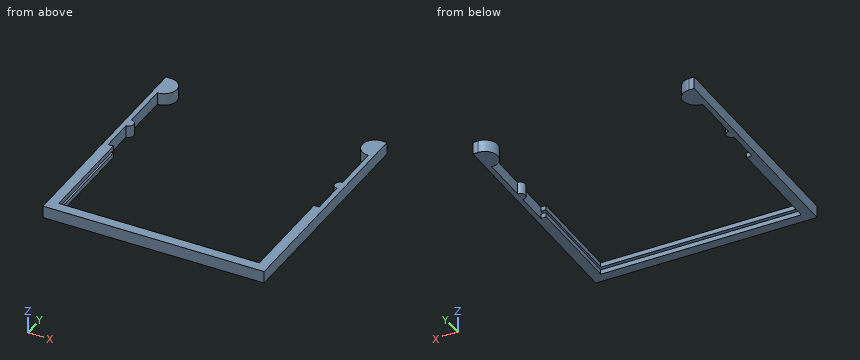
```python
from build123d import *

# Parameters (mm, degrees)
BOSS_EXTRUDE1_DEPTH      = 3
BOSS_EXTRUDE1_DEPTH_BACK = 3
CUT_EXTRUDE1_DEPTH       = 0.7
CUT_EXTRUDE1_DEPTH_BACK  = 0.7


with BuildPart() as part:
    # Sketch2 → Boss-Extrude1 (new body, two sides)
    with BuildSketch(Plane.XY) as boss_extrude1_sk:
        with BuildLine():
            Line((-52.1, 67.96), (-54.61, 67.96))
            Line((-54.61, 67.96), (-54.61, 9.929230009))
            Line((-54.61, 9.929230009), (-54.61, -46.34))
            Line((-54.61, -46.34), (54.61, -46.34))
            Line((54.61, -46.34), (54.61, 9.929230009))
            Line((54.61, 9.929230009), (54.61, 67.96))
            Line((54.61, 67.96), (52.1, 67.96))
            ThreePointArc((52.1, 67.96), (45.75, 61.61), (52.1, 55.26))
            Line((52.1, 55.26), (52.1, 43.8))
            Line((52.1, 43.8), (52.1, 31.2))
            ThreePointArc((52.1, 31.2), (49.6, 28.7), (52.1, 26.2))
            Line((52.1, 26.2), (52.1, 9.54))
            Line((52.1, 9.54), (49.53, 9.54))
            Line((49.53, 9.54), (49.53, -41.26))
            Line((49.53, -41.26), (-49.53, -41.26))
            Line((-49.53, -41.26), (-49.53, 9.54))
            Line((-49.53, 9.54), (-52.1, 9.54))
            Line((-52.1, 9.54), (-52.1, 26.2))
            ThreePointArc((-52.1, 26.2), (-49.6, 28.7), (-52.1, 31.2))
            Line((-52.1, 31.2), (-52.1, 43.8))
            Line((-52.1, 43.8), (-52.1, 55.26))
            ThreePointArc((-52.1, 55.26), (-45.75, 61.61), (-52.1, 67.96))
        make_face()
    extrude(amount=BOSS_EXTRUDE1_DEPTH)
    extrude(boss_extrude1_sk.sketch, amount=-BOSS_EXTRUDE1_DEPTH_BACK)

    # Sketch3 → Cut-Extrude1 (cut, two sides)
    with BuildSketch(Plane.XY) as cut_extrude1_sk:
        Polygon((-52.1, 9.54), (-52.1, -43.8), (52.1, -43.8), (52.1, 9.54), (49.53, 9.54), (-49.53, 9.54), align=None)
    extrude(amount=CUT_EXTRUDE1_DEPTH, mode=Mode.SUBTRACT)
    extrude(cut_extrude1_sk.sketch, amount=-CUT_EXTRUDE1_DEPTH_BACK, mode=Mode.SUBTRACT)


solid = part.part
```
Part model, mm, in its own coordinate system. Round coordinates to 2 decimals unless told otherwise and drop trailing zeros. Write each loop counter-clockwise with the first axis right and the second up, starting at its lowest first coordinate (ties: lowest second). Pieces come first, ordered by that corner, then holes. Notation, with made-up numbers: (-36, 3) -> (-5, 3) arc R19 cw to (-5, 23) -> close; hole circle Ø5 at (-20, 81). An arc over 180 degrees is marked (long way). Return JSON: item names as keys, results as strings. Group by question number.
Q1. Saw through at C-C on z = -2. Write the cut outline in (x, y).
Q2. Saw through at A-A on y = 61.61. Write the cut outline in (x, z).
Q3. Probe L1, parallel to X at y = 8, z = 2.45; L2, parallel to X at y = 61, z = -0.1; L3, parallel to Y at x = -5, z = 2.7. List the from-to ranges inside material, lowest first. Write a range as [from, to].
Q4. Pin check, flat tips, straight feed: pin 1 (1.8 mm diameter, centred on x = 6.5, z = -1.5, fed in from +Y); pin 2 (0.7 mm diameter, centred on x = 50.5, z = -1.5, fed in from +Y); pin 3 (1.2 mm diameter, centred on x = 50.5, z = 1.5, fed in from +Y). Stop position of each tip, or through.
Q5. Saw through at B-B on x = -36. Write the cut outline in (y, z).
Q6. Saw through at D-D on y = 46.5. Write the cut outline in (x, z).
Answer:
{
 "1": {"outline": "(-54.61, -46.34) -> (54.61, -46.34) -> (54.61, 67.96) -> (52.1, 67.96) arc R6.35 ccw to (52.1, 55.26) -> (52.1, 31.2) arc R2.5 ccw to (52.1, 26.2) -> (52.1, 9.54) -> (49.53, 9.54) -> (49.53, -41.26) -> (-49.53, -41.26) -> (-49.53, 9.54) -> (-52.1, 9.54) -> (-52.1, 26.2) arc R2.5 ccw to (-52.1, 31.2) -> (-52.1, 55.26) arc R6.35 ccw to (-52.1, 67.96) -> (-54.61, 67.96) -> close"},
 "2": {"outline": "(-54.61, -3) -> (-45.75, -3) -> (-45.75, 3) -> (-54.61, 3) -> close; (45.75, -3) -> (54.61, -3) -> (54.61, 3) -> (45.75, 3) -> close"},
 "3": {"L1": "[-54.61, -49.53], [49.53, 54.61]", "L2": "[-54.61, -45.78], [45.78, 54.61]", "L3": "[-46.34, -41.26]"},
 "4": {"pin 1": "y = -41.26", "pin 2": "y = 67.84", "pin 3": "y = 67.88"},
 "5": {"outline": "(-46.34, -3) -> (-41.26, -3) -> (-41.26, -0.7) -> (-43.8, -0.7) -> (-43.8, 0.7) -> (-41.26, 0.7) -> (-41.26, 3) -> (-46.34, 3) -> close"},
 "6": {"outline": "(-54.61, -3) -> (-52.1, -3) -> (-52.1, 3) -> (-54.61, 3) -> close; (52.1, -3) -> (54.61, -3) -> (54.61, 3) -> (52.1, 3) -> close"}
}
